Model file for the job. Use its own axes, mm. Give positions to 0.01 mm unless a question says otherwise; leave off trailing zeros. Loops run counter-clockwise (first coordinate to the right, second up) from the corner with the lowest first, then second, coordinate; pieces in that order, holes last. Notation, with made-up numbers: M 21.5,83 L 35.5,83 A25 ccw 35.5,95 Z; hole C 6.5,21 d4. An arc over 180 degrees is marked long. Answer in a Markdown table with one row per item.
```python
from build123d import *

# Parameters (mm, degrees)
BASE_DEPTH                = 5
ESQUISSE3_R               = 2
ESQUISSE3_W               = 65
ESQUISSE3_H               = 30
ENL_V_MAT_EXTRU_1_DEPTH   = 6
CONG_1_R                  = 3
PER_AGE_POUR_BILLES_REACH = 7
ESQUISSE6_R               = 2
ESQUISSE6_R_2             = 11
PER_AGE_POUR_PROFIL_REACH = 7
ESQUISSE8_R               = 3
ESQUISSE13_R              = 2
ENL_V_MAT_EXTRU_4_DEPTH   = 10
ESQUISSE14_R              = 2
ENL_V_MAT_EXTRU_5_DEPTH   = 10


with BuildPart() as part:
    # Esquisse1 → Base (new body)
    with BuildSketch(Plane.XY):
        Polygon((0, 0), (-175, 0), (-199.748737342, 24.748737342), (-199.748737342, 247.248737342), (-175, 271.997474683), (0, 271.997474683), (24.748737342, 247.248737342), (24.748737342, 24.748737342), align=None)
    extrude(amount=BASE_DEPTH)

    # Esquisse3 → Enlèv. mat.-Extru.1 (cut, through all)
    with BuildSketch(Plane(origin=(0, 0, 0), x_dir=(-1, 0, 0), z_dir=(0, 0, -1))):
        with Locations((52.5, 45)):
            Circle(ESQUISSE3_R)
        with Locations((122.5, 45)):
            Circle(ESQUISSE3_R)
        with Locations((122.5, 226.997474683)):
            Circle(ESQUISSE3_R)
        with Locations((52.5, 226.997474683)):
            Circle(ESQUISSE3_R)
        Polygon((129.5, 0), (129.5, 20), (105.5, 20), (105.5, 45.5), (69.5, 45.5), (69.5, 20), (45.5, 20), (45.5, 0), align=None)
        Polygon((45.5, 271.997474683), (129.5, 271.997474683), (129.5, 251.997474683), (105.5, 251.997474683), (105.5, 226.497474683), (69.5, 226.497474683), (69.5, 251.997474683), (45.5, 251.997474683), align=None)
        with Locations((87.5, 201.997474683)):
            Rectangle(ESQUISSE3_W, ESQUISSE3_H)
        with Locations((87.5, 70)):
            Rectangle(ESQUISSE3_W, ESQUISSE3_H)
    extrude(amount=-ENL_V_MAT_EXTRU_1_DEPTH, mode=Mode.SUBTRACT)

    # Congé1
    cong_1_edges = [part.edges().sort_by_distance(p)[0] for p in [
        (0, 0, 2.5),
        (-175, 0, 2.5),
        (-199.748737342, 24.748737342, 2.5),
        (-199.748737342, 247.248737342, 2.5),
        (-175, 271.997474683, 2.5),
        (0, 271.997474683, 2.5),
        (24.748737342, 247.248737342, 2.5),
        (24.748737342, 24.748737342, 2.5),
        (-45.5, 251.997474683, 2.5),
        (-45.5, 271.997474683, 2.5),
        (-129.5, 271.997474683, 2.5),
        (-129.5, 251.997474683, 2.5),
        (-105.5, 251.997474683, 2.5),
        (-105.5, 226.497474683, 2.5),
        (-69.5, 226.497474683, 2.5),
        (-69.5, 251.997474683, 2.5),
        (-129.5, 0, 2.5),
        (-45.5, 0, 2.5),
        (-45.5, 20, 2.5),
        (-69.5, 20, 2.5),
        (-69.5, 45.5, 2.5),
        (-105.5, 45.5, 2.5),
        (-105.5, 20, 2.5),
        (-129.5, 20, 2.5),
    ]]
    fillet(cong_1_edges, radius=CONG_1_R)

    # Esquisse6 → Perçage pour billes (cut, up to next)
    with BuildSketch(Plane.XY.offset(5), mode=Mode.PRIVATE) as per_age_pour_billes_sk1:
        with Locations((-1.784271247, 16)):
            Circle(ESQUISSE6_R)
    per_age_pour_billes_tool1 = extrude(per_age_pour_billes_sk1.sketch, amount=-PER_AGE_POUR_BILLES_REACH, mode=Mode.PRIVATE) & part.part
    add(per_age_pour_billes_tool1.solids().sort_by_distance((-1.784271, 16, 5))[0], mode=Mode.SUBTRACT)
    # Esquisse6 → Perçage pour billes (cut, up to next)
    with BuildSketch(Plane.XY.offset(5), mode=Mode.PRIVATE) as per_age_pour_billes_sk2:
        with Locations((-1.784271247, 46)):
            Circle(ESQUISSE6_R)
    per_age_pour_billes_tool2 = extrude(per_age_pour_billes_sk2.sketch, amount=-PER_AGE_POUR_BILLES_REACH, mode=Mode.PRIVATE) & part.part
    add(per_age_pour_billes_tool2.solids().sort_by_distance((-1.784271, 46, 5))[0], mode=Mode.SUBTRACT)
    # Esquisse6 → Perçage pour billes (cut, up to next)
    with BuildSketch(Plane.XY.offset(5), mode=Mode.PRIVATE) as per_age_pour_billes_sk3:
        with Locations((-1.784271247, 225.997474683)):
            Circle(ESQUISSE6_R)
    per_age_pour_billes_tool3 = extrude(per_age_pour_billes_sk3.sketch, amount=-PER_AGE_POUR_BILLES_REACH, mode=Mode.PRIVATE) & part.part
    add(per_age_pour_billes_tool3.solids().sort_by_distance((-1.784271, 225.997475, 5))[0], mode=Mode.SUBTRACT)
    # Esquisse6 → Perçage pour billes (cut, up to next)
    with BuildSketch(Plane.XY.offset(5), mode=Mode.PRIVATE) as per_age_pour_billes_sk4:
        with Locations((-1.784271247, 255.997474683)):
            Circle(ESQUISSE6_R)
    per_age_pour_billes_tool4 = extrude(per_age_pour_billes_sk4.sketch, amount=-PER_AGE_POUR_BILLES_REACH, mode=Mode.PRIVATE) & part.part
    add(per_age_pour_billes_tool4.solids().sort_by_distance((-1.784271, 255.997475, 5))[0], mode=Mode.SUBTRACT)
    # Esquisse6 → Perçage pour billes (cut, up to next)
    with BuildSketch(Plane.XY.offset(5), mode=Mode.PRIVATE) as per_age_pour_billes_sk5:
        with Locations((-1.784271247, 240.997474683)):
            Circle(ESQUISSE6_R_2)
    per_age_pour_billes_tool5 = extrude(per_age_pour_billes_sk5.sketch, amount=-PER_AGE_POUR_BILLES_REACH, mode=Mode.PRIVATE) & part.part
    add(per_age_pour_billes_tool5.solids().sort_by_distance((-1.784271, 240.997475, 5))[0], mode=Mode.SUBTRACT)
    # Esquisse6 → Perçage pour billes (cut, up to next)
    with BuildSketch(Plane.XY.offset(5), mode=Mode.PRIVATE) as per_age_pour_billes_sk6:
        with Locations((-1.784271247, 31)):
            Circle(ESQUISSE6_R_2)
    per_age_pour_billes_tool6 = extrude(per_age_pour_billes_sk6.sketch, amount=-PER_AGE_POUR_BILLES_REACH, mode=Mode.PRIVATE) & part.part
    add(per_age_pour_billes_tool6.solids().sort_by_distance((-1.784271, 31, 5))[0], mode=Mode.SUBTRACT)
    # Esquisse6 → Perçage pour billes (cut, up to next)
    with BuildSketch(Plane.XY.offset(5), mode=Mode.PRIVATE) as per_age_pour_billes_sk7:
        with Locations((-173.215728753, 16)):
            Circle(ESQUISSE6_R)
    per_age_pour_billes_tool7 = extrude(per_age_pour_billes_sk7.sketch, amount=-PER_AGE_POUR_BILLES_REACH, mode=Mode.PRIVATE) & part.part
    add(per_age_pour_billes_tool7.solids().sort_by_distance((-173.215729, 16, 5))[0], mode=Mode.SUBTRACT)
    # Esquisse6 → Perçage pour billes (cut, up to next)
    with BuildSketch(Plane.XY.offset(5), mode=Mode.PRIVATE) as per_age_pour_billes_sk8:
        with Locations((-173.215728753, 46)):
            Circle(ESQUISSE6_R)
    per_age_pour_billes_tool8 = extrude(per_age_pour_billes_sk8.sketch, amount=-PER_AGE_POUR_BILLES_REACH, mode=Mode.PRIVATE) & part.part
    add(per_age_pour_billes_tool8.solids().sort_by_distance((-173.215729, 46, 5))[0], mode=Mode.SUBTRACT)
    # Esquisse6 → Perçage pour billes (cut, up to next)
    with BuildSketch(Plane.XY.offset(5), mode=Mode.PRIVATE) as per_age_pour_billes_sk9:
        with Locations((-173.215728753, 31)):
            Circle(ESQUISSE6_R_2)
    per_age_pour_billes_tool9 = extrude(per_age_pour_billes_sk9.sketch, amount=-PER_AGE_POUR_BILLES_REACH, mode=Mode.PRIVATE) & part.part
    add(per_age_pour_billes_tool9.solids().sort_by_distance((-173.215729, 31, 5))[0], mode=Mode.SUBTRACT)
    # Esquisse6 → Perçage pour billes (cut, up to next)
    with BuildSketch(Plane.XY.offset(5), mode=Mode.PRIVATE) as per_age_pour_billes_sk10:
        with Locations((-173.215728753, 225.997474683)):
            Circle(ESQUISSE6_R)
    per_age_pour_billes_tool10 = extrude(per_age_pour_billes_sk10.sketch, amount=-PER_AGE_POUR_BILLES_REACH, mode=Mode.PRIVATE) & part.part
    add(per_age_pour_billes_tool10.solids().sort_by_distance((-173.215729, 225.997475, 5))[0], mode=Mode.SUBTRACT)
    # Esquisse6 → Perçage pour billes (cut, up to next)
    with BuildSketch(Plane.XY.offset(5), mode=Mode.PRIVATE) as per_age_pour_billes_sk11:
        with Locations((-173.215728753, 255.997474683)):
            Circle(ESQUISSE6_R)
    per_age_pour_billes_tool11 = extrude(per_age_pour_billes_sk11.sketch, amount=-PER_AGE_POUR_BILLES_REACH, mode=Mode.PRIVATE) & part.part
    add(per_age_pour_billes_tool11.solids().sort_by_distance((-173.215729, 255.997475, 5))[0], mode=Mode.SUBTRACT)
    # Esquisse6 → Perçage pour billes (cut, up to next)
    with BuildSketch(Plane.XY.offset(5), mode=Mode.PRIVATE) as per_age_pour_billes_sk12:
        with Locations((-173.215728753, 240.997474683)):
            Circle(ESQUISSE6_R_2)
    per_age_pour_billes_tool12 = extrude(per_age_pour_billes_sk12.sketch, amount=-PER_AGE_POUR_BILLES_REACH, mode=Mode.PRIVATE) & part.part
    add(per_age_pour_billes_tool12.solids().sort_by_distance((-173.215729, 240.997475, 5))[0], mode=Mode.SUBTRACT)

    # Esquisse8 → Perçage pour profilé (cut, up to next)
    with BuildSketch(Plane.XY.offset(5), mode=Mode.PRIVATE) as per_age_pour_profil_sk1:
        with Locations((-152.5, 23)):
            Circle(ESQUISSE8_R)
    per_age_pour_profil_tool1 = extrude(per_age_pour_profil_sk1.sketch, amount=-PER_AGE_POUR_PROFIL_REACH, mode=Mode.PRIVATE) & part.part
    add(per_age_pour_profil_tool1.solids().sort_by_distance((-152.5, 23, 5))[0], mode=Mode.SUBTRACT)
    # Esquisse8 → Perçage pour profilé (cut, up to next)
    with BuildSketch(Plane.XY.offset(5), mode=Mode.PRIVATE) as per_age_pour_profil_sk2:
        with Locations((-152.5, 248.997474683)):
            Circle(ESQUISSE8_R)
    per_age_pour_profil_tool2 = extrude(per_age_pour_profil_sk2.sketch, amount=-PER_AGE_POUR_PROFIL_REACH, mode=Mode.PRIVATE) & part.part
    add(per_age_pour_profil_tool2.solids().sort_by_distance((-152.5, 248.997475, 5))[0], mode=Mode.SUBTRACT)
    # Esquisse8 → Perçage pour profilé (cut, up to next)
    with BuildSketch(Plane.XY.offset(5), mode=Mode.PRIVATE) as per_age_pour_profil_sk3:
        with Locations((-22.5, 248.997474683)):
            Circle(ESQUISSE8_R)
    per_age_pour_profil_tool3 = extrude(per_age_pour_profil_sk3.sketch, amount=-PER_AGE_POUR_PROFIL_REACH, mode=Mode.PRIVATE) & part.part
    add(per_age_pour_profil_tool3.solids().sort_by_distance((-22.5, 248.997475, 5))[0], mode=Mode.SUBTRACT)
    # Esquisse8 → Perçage pour profilé (cut, up to next)
    with BuildSketch(Plane.XY.offset(5), mode=Mode.PRIVATE) as per_age_pour_profil_sk4:
        with Locations((-22.5, 23)):
            Circle(ESQUISSE8_R)
    per_age_pour_profil_tool4 = extrude(per_age_pour_profil_sk4.sketch, amount=-PER_AGE_POUR_PROFIL_REACH, mode=Mode.PRIVATE) & part.part
    add(per_age_pour_profil_tool4.solids().sort_by_distance((-22.5, 23, 5))[0], mode=Mode.SUBTRACT)

    # Esquisse13 → Enlèv. mat.-Extru.4 (cut)
    with BuildSketch(Plane.XY.offset(5)):
        with Locations((-20.251262658, 185.998737342)):
            Circle(ESQUISSE13_R)
        with Locations((-20.251262658, 165.998737342)):
            Circle(ESQUISSE13_R)
        with Locations((-20.251262658, 105.998737342)):
            Circle(ESQUISSE13_R)
        with Locations((-20.251262658, 85.998737342)):
            Circle(ESQUISSE13_R)
    extrude(amount=-ENL_V_MAT_EXTRU_4_DEPTH, mode=Mode.SUBTRACT)

    # Esquisse14 → Enlèv. mat.-Extru.5 (cut)
    with BuildSketch(Plane.XY.offset(5)):
        with Locations((-120, 176.997474683)):
            Circle(ESQUISSE14_R)
        with Locations((-55, 176.997474683)):
            Circle(ESQUISSE14_R)
        with Locations((-120, 150.997474683)):
            Circle(ESQUISSE14_R)
        with Locations((-55, 150.997474683)):
            Circle(ESQUISSE14_R)
        with Locations((-120, 121)):
            Circle(ESQUISSE14_R)
        with Locations((-55, 121)):
            Circle(ESQUISSE14_R)
        with Locations((-55, 95)):
            Circle(ESQUISSE14_R)
        with Locations((-120, 95)):
            Circle(ESQUISSE14_R)
    extrude(amount=-ENL_V_MAT_EXTRU_5_DEPTH, mode=Mode.SUBTRACT)


solid = part.part
```
Q1. Saw through at D-D (x = -152.5). Give the cut face in (y, z), and give its area (3 significant figures).
Reported:
| item | result |
|---|---|
| outline | M 0,0 L 20,0 L 20,5 L 0,5 Z; M 26,0 L 246,0 L 246,5 L 26,5 Z; M 252,0 L 272,0 L 272,5 L 252,5 Z |
| area | 1,300 mm² |
Q2. Mould opens along X. For faces 1 (the face through (-4.17, 230.26, 2.54)), 2 (the face through (-187, 12, 2)), 3 (the face through (12, 260, 2)) say: released by +X, released by -X, zero draft, split by the parting line, or undercut.
Reported:
| item | result |
|---|---|
| face 1 | undercut |
| face 2 | released by -X |
| face 3 | released by +X |
Q3. Probe probe 1 along Y at (x, z) = (-102, 4.2); probe 2 along Y at (x, z) = (-152.5, 3.75); probe 3 along X at (y, z) = (94, 1.9). List the from-to ranges inside material, lowest first.
Reported:
| item | result |
|---|---|
| probe 1 | 45.5 to 55, 85 to 187, 217 to 226.5 |
| probe 2 | 0 to 20, 26 to 246, 252 to 272 |
| probe 3 | -199.75 to -121.73, -118.27 to -56.73, -53.27 to 24.75 |
Q4. Saw through at C-C (y = 31). Give the cut face in (x, z).
Reported:
| item | result |
|---|---|
| outline | M -199.75,0 L -184.22,0 L -184.22,5 L -199.75,5 Z; M -162.22,0 L -105.5,0 L -105.5,5 L -162.22,5 Z; M -69.5,0 L -12.78,0 L -12.78,5 L -69.5,5 Z; M 9.22,0 L 24.75,0 L 24.75,5 L 9.22,5 Z |
Q5. Saw through at B-B (x = -89). Give the cut face in (y, z), and give its area (3 significant figures).
Reported:
| item | result |
|---|---|
| outline | M 45.5,0 L 55,0 L 55,5 L 45.5,5 Z; M 85,0 L 187,0 L 187,5 L 85,5 Z; M 217,0 L 226.5,0 L 226.5,5 L 217,5 Z |
| area | 605 mm² |
Q6. Saw through at A-A (y = 209). Give the cut face in (x, z).
Reported:
| item | result |
|---|---|
| outline | M -199.75,0 L -120,0 L -120,5 L -199.75,5 Z; M -55,0 L 24.75,0 L 24.75,5 L -55,5 Z |
Q7. Drop flat-ended pins along their axis: pin 1 (3 mm diameter, centred on x = -173.22, y = 46, fed in from -Z); pin 2 (2.5 mm diameter, centred on y = 259.5, z = 1.5, fed in from -X). Give the stop position or say it passes through.
Reported:
| item | result |
|---|---|
| pin 1 | through |
| pin 2 | x = -188.75 |
